The model under review builds one solid part; all positions refer to its coordinate system, in mm. A direction names the side the tool comes from. Coordinates: 2 decimals unless noted, no trailing zeros. Order: outer loops, then holes, each group sorted by start corner. A loop starts at its lowest first (then second) coordinate and runs counter-clockwise, first axis right, second up. Notation, with made-up numbers: M -14,-24.5 L 5,-24.5 A21 cw 5,-17.5 Z; hole C 86.25,-30.5 d6. An arc over 180 degrees is marked long. Write each question's results on one line, items separated by ' | '.
from build123d import *

# Parameters (mm, degrees)
PATTERN_CIRCULAR_1_COUNT = 4
PATTERN_CIRCULAR_1_ANGLE = 180
CUT_EXTRUDE_1_DEPTH      = 63.425956281


with BuildPart() as part:
    # Эскиз1 → Повернуть1 (revolve)
    with BuildSketch(Plane(origin=(0, 0, 0), x_dir=(0, 0, -1), z_dir=(1, 0, 0))):
        with BuildLine():
            Line((0, 0), (44, 0))
            Line((44, 0), (44, 4))
            ThreePointArc((44, 4), (43.707106781, 4.707106781), (43, 5))
            Line((43, 5), (0, 5))
            Line((0, 5), (0, 0))
        make_face()
    revolve(axis=Axis((0, 0, 0), (0, 1, 0)))

    # Эскиз2 → Вырез-Повернуть1 (revolve, cut)
    with BuildSketch(Plane(origin=(0, 0, 0), x_dir=(0, 0, -1), z_dir=(1, 0, 0))):
        Polygon((-39, 0), (-37.5, 0), (-37.5, 3), (-37, 3), (-37, 5), (-39, 5), align=None)
    cut_revolve_1 = revolve(axis=Axis((0, 0, 39), (0, 1, 0)), mode=Mode.SUBTRACT)

    # Круговой массив1: Вырез-Повернуть1 ×4 about axis
    pattern_circular_1_axis = Axis((0, 0, 0), (0, -1, 0))
    for i in range(1, PATTERN_CIRCULAR_1_COUNT):
        add(cut_revolve_1.rotate(pattern_circular_1_axis, i * PATTERN_CIRCULAR_1_ANGLE / (PATTERN_CIRCULAR_1_COUNT - 1)), mode=Mode.SUBTRACT)

    # Эскиз3 → Вырез-Вытянуть1 (cut, through all)
    with BuildSketch(Plane.XZ):
        with BuildLine():
            Line((32.759496508, 29.373719352), (32.759496508, -29.373719352))
            ThreePointArc((32.759496508, -29.373719352), (44, 0), (32.759496508, 29.373719352))
        make_face()
    extrude(amount=-CUT_EXTRUDE_1_DEPTH, mode=Mode.SUBTRACT)


solid = part.part
1) For pin 1 (2 mm diameter, centred on y = 0.5, z = 22, fed in from -X); pin 2 (3 mm diameter, centred on x = -0.5, z = -38, fed in from +Y); pin 3 (3 mm diameter, centred on x = 20.5, y = 2.5, fed in from +Z); pin 4 (1.8 mm diameter, centred on x = 0, z = 39, fed in from +Y), all flat-tipped, find the tip position at first contact; note any pin that passes through.
Solutions:
pin 1: x = -38.67 | pin 2: y = 5 | pin 3: z = 39.69 | pin 4: through
2) The part is to be moulded in two halves that separate along Z. For faces 3 (the flat face through (-6, 5, 1)), 4 (the cylindrical face through (-43.975, 2.028, -1.485)), 5 (the cylindrical face through (-34.4, 4, -21.4)), say which applies: pulls with the +Z half, pulls with the -Z half, needs draft (parallel to the pull), parting line crosses it, or undercut.
Solutions:
face 3: needs draft | face 4: parting line crosses it | face 5: undercut
3) For faces 1 (the cylindrical face through (-0.9, 1.5, -40.2)), 2 (the flat face through (-33, 3, -21)), list the 3-axis set-ups (+Z, -Z, +X, -X, +Y, -Y) from which the entire face can be reached by the end or side of a thin tool; tool diameter is ignored.
Solutions:
face 1: +Y, -Y | face 2: +Y
4) Take a section at B-B on y = 1.05. Count the separate pieces of the cut face and the enclosed holes in it, plus the area to 3 significant figures.
Solutions:
separate pieces: 1 | enclosed holes: 4 | area: 5,600 mm2
5) Take a section at A-A on x = 0. State the section outline as (y, z) points.
Solutions:
outline: M 0,-44 L 4,-44 A1 ccw 5,-43 L 5,-41 L 3,-41 L 3,-40.5 L 0,-40.5 Z; M 0,-37.5 L 3,-37.5 L 3,-37 L 5,-37 L 5,37 L 3,37 L 3,37.5 L 0,37.5 Z; M 0,40.5 L 3,40.5 L 3,41 L 5,41 L 5,43 A1 ccw 4,44 L 0,44 Z
6) To check wall thickness, follow line 1 along Z through (x, y) = (0, 1.5); line 2 along Z through (x, y) = (-33, 2.5); line 3 along Z through (x, y) = (-15, 4.75). State the ranges of each line that lie inside material, in increasing order.
Solutions:
line 1: -44 to -40.5, -37.5 to 37.5, 40.5 to 44 | line 2: -29.1 to -20.78, -18.22 to 18.22, 20.78 to 29.1 | line 3: -41 to 41
